```python
from build123d import *

# Parameters (mm, degrees)
EXTRUDE_1_DEPTH     = 65
FILLET_1_R          = 2
SKETCH_2_W          = 4
SKETCH_2_H          = 8
CUT_EXTRUDE_1_DEPTH = 4
SKETCH_4_W          = 4
SKETCH_4_H          = 4
EXTRUDE_2_DEPTH     = 7
SKETCH_5_R          = 0.5
EXTRUDE_3_DEPTH     = 5


with BuildPart() as part:
    # Эскиз1 → Бобышка-Вытянуть1 (new body)
    with BuildSketch(Plane.XY):
        with BuildLine():
            Line((32.5, -9.5), (-32.5, -9.5))
            ThreePointArc((-32.5, -9.5), (-33.914213562, -8.914213562), (-34.5, -7.5))
            Line((-34.5, -7.5), (-34.5, 7.5))
            ThreePointArc((-34.5, 7.5), (-33.914213562, 8.914213562), (-32.5, 9.5))
            Line((-32.5, 9.5), (32.5, 9.5))
            ThreePointArc((32.5, 9.5), (33.914213562, 8.914213562), (34.5, 7.5))
            Line((34.5, 7.5), (34.5, -7.5))
            ThreePointArc((34.5, -7.5), (33.914213562, -8.914213562), (32.5, -9.5))
        make_face()
    extrude(amount=EXTRUDE_1_DEPTH)

    # Скругление1
    fillet_1_edges = [part.edges().sort_by_distance(p)[0] for p in [
        (-33.914213562, -8.914213562, 65),
        (-34.5, 0, 0),
        (-33.914213562, 8.914213562, 0),
        (0, -9.5, 65),
        (33.914213562, -8.914213562, 65),
        (34.5, 0, 65),
        (33.914213562, 8.914213562, 65),
        (0, 9.5, 65),
        (-33.914213562, 8.914213562, 65),
        (-34.5, 0, 65),
        (0, 9.5, 0),
        (33.914213562, 8.914213562, 0),
        (34.5, 0, 0),
        (33.914213562, -8.914213562, 0),
        (0, -9.5, 0),
        (-33.914213562, -8.914213562, 0),
    ]]
    fillet(fillet_1_edges, radius=FILLET_1_R)

    # Эскиз2 → Вырез-Вытянуть1 (cut)
    with BuildSketch(Plane(origin=(0, 9.5, 0), x_dir=(1, 0, 0), z_dir=(0, 1, 0))):
        with Locations((-27.5, -12)):
            Rectangle(SKETCH_2_W, SKETCH_2_H)
    extrude(amount=-CUT_EXTRUDE_1_DEPTH, mode=Mode.SUBTRACT)

    # Эскиз4 → Бобышка-Вытянуть2 (add)
    with BuildSketch(Plane(origin=(0, 5.5, 0), x_dir=(1, 0, 0), z_dir=(0, 1, 0))):
        with Locations((-27.5, -10)):
            Rectangle(SKETCH_4_W, SKETCH_4_H)
    extrude(amount=EXTRUDE_2_DEPTH)

    # Эскиз5 → Бобышка-Вытянуть3 (add)
    with BuildSketch(Plane.ZY.offset(34.5)):
        with Locations(Location((55, 0, 0), (0, 0, 180))):
            Circle(SKETCH_5_R)
        with Locations(Location((57, 0, 0), (0, 0, 180))):
            Circle(SKETCH_5_R)
    extrude(amount=EXTRUDE_3_DEPTH)


solid = part.part
```
Geometry: final body of the model. Coordinates: model frame, mm. A direction names the side the tool comes from. Round coordinates to 2 decimals unless told otherwise and drop trailing zeros. Loops run counter-clockwise (first coordinate to the right, second up) from the corner with the lowest first, then second, coordinate; pieces in that order, holes last.
Item 1: Section B-B, the plane y = 2.5. Output: boundary loops of the cut face in (x, z), plus the area to 3 significant figures.
Checked values:
outline: (-34.5, 2) arc R2 ccw to (-32.5, 0) - (32.5, 0) arc R2 ccw to (34.5, 2) - (34.5, 63) arc R2 ccw to (32.5, 65) - (-32.5, 65) arc R2 ccw to (-34.5, 63) - close
area: 4,480 mm2
Item 2: Line query: L1, parallel to Y at x = -28, z = 7; L2, parallel to Z at x = -26, y = 7.75; L3, parallel to X at y = 7, z = 11. Output: solid intervals per line, ascending.
Checked values:
L1: y = -9.5 to 9.5
L2: z = 0.02 to 12, 16 to 64.98
L3: x = -34.5 to 34.5
Item 3: Reachability of faces 4 (the flat face through (-28, 5.5, 14)), 5 (the flat face through (-28, 11, 8)), 6 (the flat face through (34.5, 0, 32)) from +Z, -Z, +X, -X, +Y, -Y: full face, straight path, thin tool, end or side. Return the list, or none.
Checked values:
face 4: +Y
face 5: -Z, +X, -X, +Y
face 6: +Z, -Z, +X, +Y, -Y
Item 4: Contact query for flat-ended pins moving along their axis: P1, Ø10, axis at x = -2, z = 12.5, coming from the +Y side; P2, Ø0.9, axis at x = -28, y = 11, coming from the -Z side; P3, Ø1.2, axis at x = -27.5, y = 8.5, coming from the -Z side. Output: stop coordinate, or through.
Checked values:
P1: stops at y = 9.5
P2: stops at z = 8
P3: stops at z = 0.04
Item 5: Section C-C, the plane z = 13.5. Output: boundary loops of the cut face in (x, y).
Checked values:
outline: (-34.5, -7.5) arc R2 ccw to (-32.5, -9.5) - (32.5, -9.5) arc R2 ccw to (34.5, -7.5) - (34.5, 7.5) arc R2 ccw to (32.5, 9.5) - (-25.5, 9.5) - (-25.5, 5.5) - (-29.5, 5.5) - (-29.5, 9.5) - (-32.5, 9.5) arc R2 ccw to (-34.5, 7.5) - close
Item 6: Mould query, pull axis X, two halves, no side actions, for faces 1 (the cylindrical face through (0.45, 8.93, 0.6)), 2 (the flat face through (-25.5, 11, 10)), 3 (the flat face through (-29.5, 8, 14)). Classes: released by +X, released by -X, zero draft, split by the parting line, or undercut.
Checked values:
face 1: zero draft
face 2: released by +X
face 3: undercut
Item 7: Section A-A, the plane x = 14.5. Output: boundary loops of the cut face in (y, z), plus the area to 3 significant figures.
Checked values:
outline: (-9.5, 2) arc R2 ccw to (-7.5, 0) - (7.5, 0) arc R2 ccw to (9.5, 2) - (9.5, 63) arc R2 ccw to (7.5, 65) - (-7.5, 65) arc R2 ccw to (-9.5, 63) - close
area: 1,230 mm2
Item 8: Section D-D, the plane y = 11.25. Output: boundary loops of the cut face in (x, z), plus the area to 3 significant figures.
Checked values:
outline: (-29.5, 8) - (-25.5, 8) - (-25.5, 12) - (-29.5, 12) - close
area: 16.0 mm2
